Here's how the part is built. I have some questions about the finished solid (model axes, mm). A direction names the side the tool comes from. Give positions to 0.01 mm unless a question says otherwise; leave off trailing zeros. Write each loop counter-clockwise with the first axis right and the second up, starting at its lowest first coordinate (ties: lowest second). Pieces come first, ordered by that corner, then holes. Notation, with made-up numbers: (49.25, 6.5) - (94.25, 6.5) arc R15 cw to (94.25, 15.5) - close; hole circle Ø9 at (25, -12.5). An arc over 180 degrees is marked (long way). Use one line per item in the form item = value. Start each with the question number.
from build123d import *

# Parameters (mm, degrees)
F0_R     = 4.75
F1_DEPTH = 4.5
F2_R     = 50
F3_SIZE  = 1
F5_DEPTH = 25
F6_SIZE  = 1


with BuildPart() as f1:
    # F0 (on Top) → F1 (new body, symmetric)
    with BuildSketch(Plane.XY):
        with BuildLine():
            Line((25, 0), (8.288939, 39.506208))
            ThreePointArc((8.288939, 39.506208), (0, 45), (-8.288939, 39.506208))
            Line((-8.288939, 39.506208), (-25, 0))
            Line((-25, 0), (-8.288939, -39.506208))
            ThreePointArc((-8.288939, -39.506208), (0, -45), (8.288939, -39.506208))
            Line((8.288939, -39.506208), (25, 0))
        make_face()
        with Locations((0, -36)):
            Circle(F0_R, mode=Mode.SUBTRACT)
        with Locations((0, 36)):
            Circle(F0_R, mode=Mode.SUBTRACT)
    extrude(amount=F1_DEPTH, both=True)

    # F2
    f2_edges = [f1.edges().sort_by_distance(p)[0] for p in [
        (-25, 0, 0),
        (25, 0, 0),
    ]]
    fillet(f2_edges, radius=F2_R)

    # F3
    f3_edges = [f1.edges().sort_by_distance(p)[0] for p in [
        (0, 45, 4.5),
        (0, 45, -4.5),
        (-12.524692, -29.492569, 4.5),
        (-12.524692, -29.492569, -4.5),
    ]]
    chamfer(f3_edges, length=F3_SIZE)

    # F4 (on face) → F5 (cut)
    with BuildSketch(Plane.XY.offset(4.5)):
        Polygon((-3.525, 6.105479), (-7.05, 0), (-3.525, -6.105479), (3.525, -6.105479), (7.05, 0), (3.525, 6.105479), align=None)
    extrude(amount=-F5_DEPTH, mode=Mode.SUBTRACT)

    # F6
    f6_edges = [f1.edges().sort_by_distance(p)[0] for p in [
        (-4.75, 36, 4.5),
        (-4.75, 36, -4.5),
        (-4.75, -36, 4.5),
        (-4.75, -36, -4.5),
        (0, -6.105479, 4.5),
        (-5.2875, -3.05274, 4.5),
        (-5.2875, 3.05274, 4.5),
        (0, 6.105479, 4.5),
        (5.2875, 3.05274, 4.5),
        (5.2875, -3.05274, 4.5),
        (0, -6.105479, -4.5),
        (5.2875, -3.05274, -4.5),
        (5.2875, 3.05274, -4.5),
        (0, 6.105479, -4.5),
        (-5.2875, 3.05274, -4.5),
    ]]
    chamfer(f6_edges, length=F6_SIZE)


solid = f1.part
1. We'd pull the mould along X, two halves only. Please class faces 1 (the face through (0, 6.105, 0)), 2 (the face through (-20.71, -0.28, 0.05)), 3 (the face through (12.584, 29.352, 0.049)): pulls with the +X half, pulls with the -X half, needs draft (parallel to the pull), parting line crosses it, or undercut.
2. I want a section at C-C, the plane y = 36. List the corners of the cut face in (x, z) for me.
3. I want a section at A-A, the plane x = 0. Give the number of separate pieces and of enclosed holes in the cut face, then the cut area to 3 significant figures.
4. For faces 4 (the face through (19.87, -0.28, 4.34)), 5 (the face through (5.686, -3.349, 3.993)), 6 (the face through (5.31, 3.01, 0.05)), which set-ups out of +Z, -Z, +X, -X, +Y, -Y let a thin tool reach every point of the face, with its end or its side?
5. I want a section at B-B, the plane z = -0.5. List the corners of the cut face in (x, y) for me (3 decimals), then the cut area to 3 significant figures.
6. I want a section at D-D, the plane y = -22. List the corners of the cut face in (x, z) for me, then the cut area to 3 significant figures.
7. For P1, Ø1, axis at x = 7.5, z = 0, coming from the +Y side; P2, Ø11, axis at x = 0, y = -36, coming from the -Z side; P3, Ø5, axis at x = 1.5, z = 1.5, coming from the -Y side; P4, Ø5, axis at x = -12, z = -1.5, coming from the -Y side, each with a flat end and sliding along its axis, tell me the tip position at first contact or that it passes through.
8. Please list where these lines run through material, in increasing order: line 1 (Y direction, x = 0, z = -0.75); line 2 (Y direction, x = -1, z = -2.25); line 3 (X direction, y = -5, z = 1.5).
Result sheet:
q1.face_1 = undercut
q1.face_2 = pulls with the -X half
q1.face_3 = pulls with the +X half
q2.outline = (-9.77, -3.5) - (-8.69, -4.5) - (-5.75, -4.5) - (-4.75, -3.5) - (-4.75, 3.5) - (-5.75, 4.5) - (-8.69, 4.5) - (-9.77, 3.5) - close; (4.75, -3.5) - (5.75, -4.5) - (8.69, -4.5) - (9.77, -3.5) - (9.77, 3.5) - (8.69, 4.5) - (5.75, 4.5) - (4.75, 3.5) - close
q3.separate_pieces = 4
q3.enclosed_holes = 0
q3.area = 521 mm2
q4.face_4 = +Z, +X
q4.face_5 = +Z
q4.face_6 = +Z, -Z
q5.outline = (-16.76, -19.479) - (-8.289, -39.506) arc R9 ccw to (8.289, -39.506) - (16.76, -19.479) arc R50 ccw to (16.76, 19.479) - (8.289, 39.506) arc R9 ccw to (-8.289, 39.506) - (-16.76, 19.479) arc R50 ccw to start; hole (-7.05, 0) - (-3.525, -6.105) - (3.525, -6.105) - (7.05, 0) - (3.525, 6.105) - (-3.525, 6.105) - close; hole circle Ø9.5 at (0, -36); hole circle Ø9.5 at (0, 36)
q5.area = 2,380 mm2
q6.outline = (-15.69, -3.5) - (-14.61, -4.5) - (14.61, -4.5) - (15.69, -3.5) - (15.69, 3.5) - (14.61, 4.5) - (-14.61, 4.5) - (-15.69, 3.5) - close
q6.area = 280 mm2
q7.P1 = 41.66
q7.P2 = -4.25
q7.P3 = -45
q7.P4 = -36.64
q8.line_1 = -45 to -40.75, -31.25 to -6.11, 6.11 to 31.25, 40.75 to 45
q8.line_2 = -44.94 to -40.64, -31.36 to -6.11, 6.11 to 31.36, 40.64 to 44.94
q8.line_3 = -20.46 to -4.16, 4.16 to 20.46
